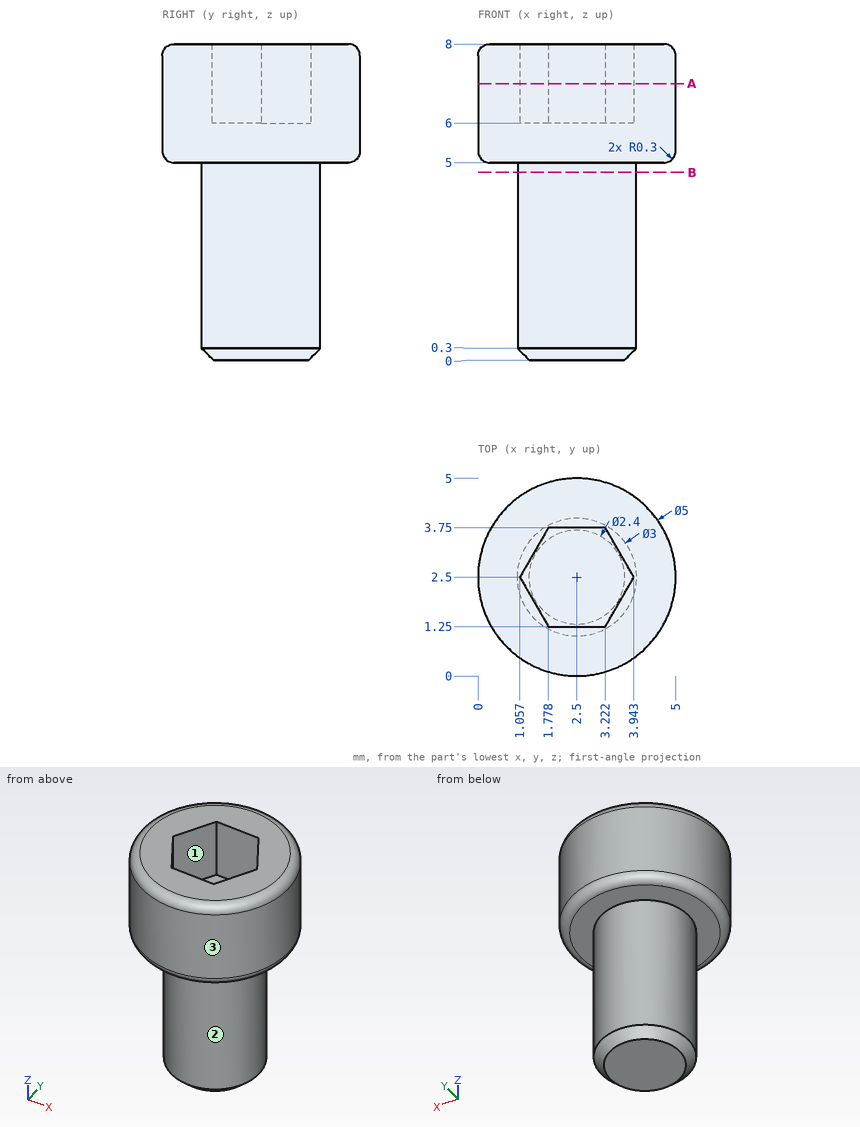
Input: dimensioned drawing with shaded views. Units: mm. Origin: part minimum x, y, z. A direction names the side the tool comes from. Give positions to 0.01 mm unless a question says otherwise; leave off trailing zeros. Write each loop counter-clockwise with the first axis right and the second up, starting at its lowest first coordinate (ties: lowest second). Pieces come first, ordered by that corner, then holes.
1. Pin query (flat end, axial travel): P1, Ø3, axis at x = 1.5, z = 1, coming from the -Y side; P2, Ø3, axis at x = 3, z = 2.5, coming from the +Y side. Return the tip coordinate at first contact, or that it passes through.
2. Section query A-A, the plane z = 7. Return loops of the section in (x, y).
3. Section query B-B, the plane z = 4.75. Return loops of the section in (x, y).
4. Line query: probe 1 along Z at (x, y) = (1.25, 1); probe 2 along Z at (x, y) = (2.1, 2.3); probe 3 along Y at (x, z) = (2.8, 7). Output: solid intervals per line, ascending.
5. Reachability of the marked faces 1, 2 and 3 from +Z, -Z, +X, -X, +Y, -Y: full face, straight path, thin tool, end or side. Return the list, or none.
Computed:
1. P1: stops at y = 1
1. P2: stops at y = 4
2. outline: circle Ø5 at (2.5, 2.5); hole (1.06, 2.5) - (1.78, 1.25) - (3.22, 1.25) - (3.94, 2.5) - (3.22, 3.75) - (1.78, 3.75) - close
3. outline: circle Ø3 at (2.5, 2.5)
4. probe 1: z = 5 to 8
4. probe 2: z = 0 to 6
4. probe 3: y = 0.02 to 1.25, 3.75 to 4.98
5. face 1: +Z
5. face 2: -Z
5. face 3: +Z, -Z
